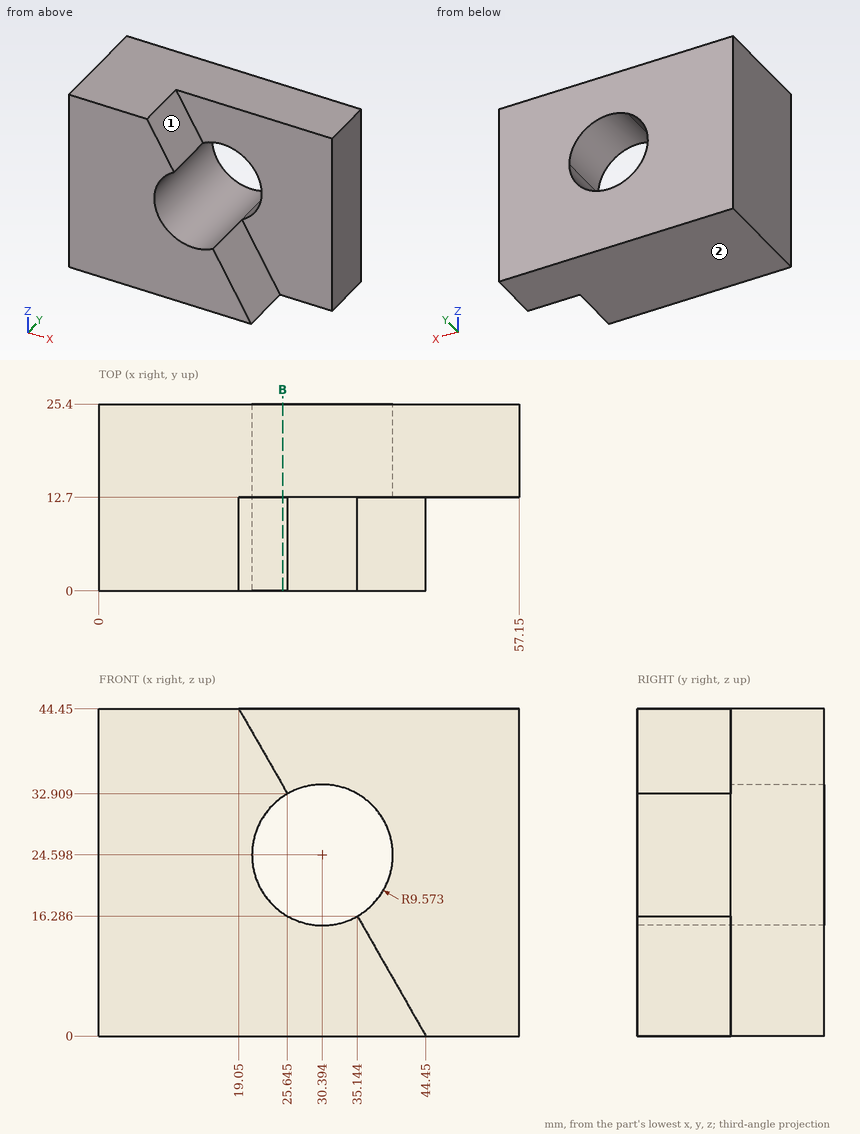
Can you work these out from the drawing? Everything is in mm from the part's minimum corner. A direction names the side the tool comes from. Give positions to 0.01 mm unless a question says otherwise; leave off trailing zeros. Write each loop counter-clockwise with the first axis right and the second up, starting at its lowest first coordinate (ties: lowest second). Pieces come first, ordered by that corner, then holes. Notation, with made-up numbers: (29.25, 61.25) -> (45.25, 61.25) arc R21 ccw to (45.25, 93.25) -> close; hole circle Ø6 at (-21.75, 77.5). An arc over 180 degrees is marked (long way). Write each question's results on one line, items separated by ' | '. Start each with the question number.
Q1. Suppose I cut it at B-B, the plane x = 25. List the corners of the cut face in (y, z) for me, and give its area (3 significant figures).
Q2. I need wall thicknesses on probe 1 along X at (y, z) = (1, 25); probe 2 along Y at (x, z) = (21, 42); probe 3 along Z at (x, y) = (27, 7) (1 decimal). Which ranges of each line are inside material? Lowest first, please.
Q3. I'm going to push flat-ended pins straight in: pin 1 Ø2 at (y, z) = (9, 29) entering from +X; pin 2 Ø10 at (y, z) = (5.5, 13) entering from +X. Where does each tip first touch, or does it pass through?
Q4. Which directions (+Z, -Z, +X, -X, +Y, -Y) give clear straight access to the entire face, cutting with the end or side of a thin tool? Please do the marked faces 1 and 2.
Outcome:
1) outline: (0, 0) -> (25.4, 0) -> (25.4, 16.69) -> (0, 16.69) -> close; (0, 32.51) -> (25.4, 32.51) -> (25.4, 44.45) -> (12.7, 44.45) -> (12.7, 34.04) -> (0, 34.04) -> close | area: 595 mm2
2) probe 1: 0 to 20.83 | probe 2: 12.7 to 25.4 | probe 3: 0 to 15.6
3) pin 1: x = 22.49 | pin 2: x = 39.88
4) face 1: +Z, +X, -Y | face 2: -Z, +X, -X, +Y, -Y
